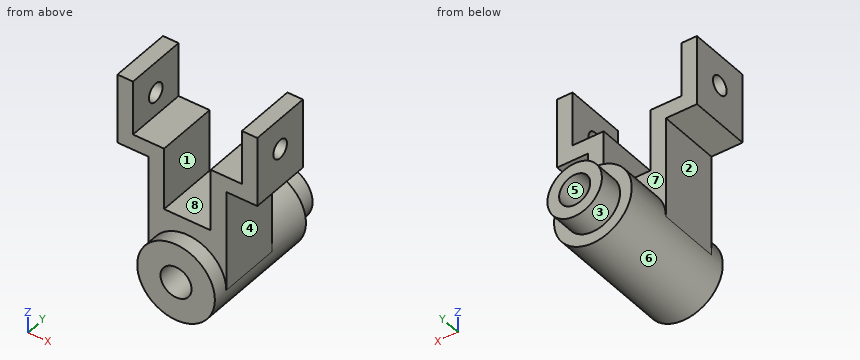
from build123d import *

# Parameters (mm, degrees)
SKETCH1_R           = 25
BOSS_EXTRUDE1_DEPTH = 80
SKETCH2_R           = 17.5
BOSS_EXTRUDE2_DEPTH = 16
SKETCH3_R           = 10
CUT_EXTRUDE1_DEPTH  = 200
BOSS_EXTRUDE3_START = 10
BOSS_EXTRUDE3_DEPTH = 40
SKETCH5_R           = 6
CUT_EXTRUDE2_DEPTH  = 100


with BuildPart() as part:
    # Sketch1 → Boss-Extrude1 (new body)
    with BuildSketch(Plane(origin=(0, 0, 0), x_dir=(1, 0, 0), z_dir=(0, 1, 0))):
        Circle(SKETCH1_R)
    extrude(amount=BOSS_EXTRUDE1_DEPTH)

    # Sketch2 → Boss-Extrude2 (add)
    with BuildSketch(Plane(origin=(0, 80, 0), x_dir=(1, 0, 0), z_dir=(0, 1, 0))):
        Circle(SKETCH2_R)
    extrude(amount=BOSS_EXTRUDE2_DEPTH)

    # Sketch3 → Cut-Extrude1 (cut)
    with BuildSketch(Plane(origin=(0, 96, 0), x_dir=(1, 0, 0), z_dir=(0, 1, 0))):
        Circle(SKETCH3_R)
    extrude(amount=-CUT_EXTRUDE1_DEPTH, mode=Mode.SUBTRACT)

    # Sketch4 → Boss-Extrude3 (add)
    with BuildSketch(Plane(origin=(0, 0, 0), x_dir=(1, 0, 0), z_dir=(0, 1, 0)).offset(BOSS_EXTRUDE3_START)):
        with BuildLine():
            Line((-25, 0), (-25, -65))
            Line((-25, -65), (-45, -65))
            Line((-45, -65), (-45, -110))
            Line((-45, -110), (-35, -110))
            Line((-35, -110), (-35, -75))
            Line((-35, -75), (-15, -75))
            Line((-15, -75), (-15, -35))
            Line((-15, -35), (0, -35))
            Line((0, -35), (15, -35))
            Line((15, -35), (15, -75))
            Line((15, -75), (35, -75))
            Line((35, -75), (35, -110))
            Line((35, -110), (45, -110))
            Line((45, -110), (45, -65))
            Line((45, -65), (25, -65))
            Line((25, -65), (25, 0))
            ThreePointArc((25, 0), (0, -25), (-25, 0))
        make_face()
    extrude(amount=BOSS_EXTRUDE3_DEPTH)

    # Sketch5 → Cut-Extrude2 (cut)
    with BuildSketch(Plane(origin=(45, 0, 0), x_dir=(0, 0, -1), z_dir=(1, 0, 0))):
        with Locations((-90, 30)):
            Circle(SKETCH5_R)
    extrude(amount=-CUT_EXTRUDE2_DEPTH, mode=Mode.SUBTRACT)


solid = part.part
The listing builds one solid part. Answer for the finished solid, in the listing's coordinates (mm). Face numbers are marked on the shaded views. A direction names the side the tool comes from. Round coordinates to 2 decimals unless told otherwise and drop trailing zeros. Write each loop counter-clockwise with the first axis right and the second up, starting at its lowest first coordinate (ties: lowest second). Pieces come first, ordered by that corner, then holes. Notation, with made-up numbers: M -27.75,33 L 1.25,33 A17 ccw 1.25,37 Z; hole C 55,-14 d8. An arc over 180 degrees is marked long. Write each question's results on one line, items separated by ' | '. Start each with the question number.
(1) The part is cut by section D-D, the plane z = -12. Write down the section's boundary in (x, y), and give its area (3 significant figures).
(2) The part is cut by section A-A, the plane y = 30. Write down the section's boundary in (x, z), and give its area (3 significant figures).
(3) The part is cut by section B-B, the plane z = 78.5. Write down the section's boundary in (x, y), and give its area (3 significant figures).
(4) Determine the mould class of the marked faces 5, 6, 7 and 8 for opening direction Z: +Z half, -Z half, draft (parallel to the pull), parting line (faces both ways), or undercut.
(5) Each of these flat-tipped pins is pushed along its axis until it touches: P1, Ø4, axis at y = 47.5, z = 17, coming from the +X side; P2, Ø22, axis at x = 23, y = 34.5, coming from the +Z side; P3, Ø4, axis at x = 10, y = 49, coming from the +Z side. Where does it stop, or does it pass through?
(6) For the marked faces 1, 2, 3 and 4, determine the directions among +Z, -Z, +X, -X, +Y, -Y from which every point of the face is accessible in a straight line to the end or side of a thin tool.
(7) The part is cut by section C-C, the plane y = 18.5. Write down the section's boundary in (x, z), and give its area (3 significant figures).
(8) Find the intervals of material crossed by line 1 (X direction, y = 19, z = 43); line 2 (Z direction, x = 0, y = 30); line 3 (Y direction, x = 39, z = 90), in increasing order.
Worked answers:
1) outline: M -21.93,0 L 21.93,0 L 21.93,80 L 12.74,80 L 12.74,96 L -12.74,96 L -12.74,80 L -21.93,80 Z | area: 3,920 mm²
2) outline: M -45,65 L -25,65 L -25,0 A25 ccw 25,0 L 25,65 L 45,65 L 45,84 L 35,84 L 35,75 L 15,75 L 15,35 L -15,35 L -15,75 L -35,75 L -35,84 L -45,84 Z; M -45,96 L -35,96 L -35,110 L -45,110 Z; M 35,96 L 45,96 L 45,110 L 35,110 Z; hole C 0,0 d20 | area: 4,080 mm²
3) outline: M -45,10 L -35,10 L -35,50 L -45,50 Z; M 35,10 L 45,10 L 45,50 L 35,50 Z | area: 800 mm²
4) face 5: undercut | face 6: parting line | face 7: draft | face 8: +Z half
5) P1: stops at x = 25 | P2: stops at z = 75 | P3: stops at z = 35
6) face 1: +Z, +Y, -Y | face 2: -Z, -X, +Y, -Y | face 3: +Y | face 4: -Z, +X, +Y, -Y
7) outline: M -45,65 L -25,65 L -25,0 A25 ccw 25,0 L 25,65 L 45,65 L 45,110 L 35,110 L 35,75 L 15,75 L 15,35 L -15,35 L -15,75 L -35,75 L -35,110 L -45,110 Z; hole C 0,0 d20 | area: 4,320 mm²
8) line 1: x = -25 to -15, 15 to 25 | line 2: z = -25 to -10, 10 to 35 | line 3: y = 10 to 24, 36 to 50
